The listing builds one solid part. Answer for the finished solid, in the listing's coordinates (mm). A direction names the side the tool comes from. Coordinates: 2 decimals unless noted, no trailing zeros. Order: outer loops, then holes, each group sorted by start corner. A loop starts at its lowest first (then second) coordinate and runs counter-clockwise, first axis right, second up. Notation, with made-up numbers: (57.5, 11) - (69.5, 11) arc R13 cw to (69.5, 19) - close; hole circle Ø3 at (1.5, 43). An arc over 180 degrees is marked (long way). Use one line per item in the form item = value. Start each with the question number.
Item 1: Each of these flat-tipped pins is pushed along its axis until it touches: pin 1 Ø3 at (x, y) = (139.5, 5.5) entering from -Z; pin 2 Ø5 at (x, y) = (48.5, 4.5) entering from -Z; pin 3 Ø4 at (x, z) = (72, 21.5) entering from +Y. Where does it stop, or does it pass through?
Item 2: Section B-B, the plane z = 2 is taken. Write down the section's boundary in (x, y).
Item 3: A tool of negligible diameter and unlimited length cuts with its end or side. For faces 4 (the flat face through (103.68, 5.07, -15)), 5 (the flat face through (137, 5, -21)), 6 (the flat face through (122.249, 5.07, -6.156)), from which of +Z, -Z, +X, -X, +Y, -Y can it reach the whole face along a straight path? Write none if from no direction.
Item 4: Section C-C, the plane x = 119.5 is taken. Write down the section's boundary in (y, z), and give its area (3 significant figures).
Item 5: The mould has two halves that part along Y. Classify faces 1 (the cylindrical face through (75.707, 5.066, 12.856)), 2 (the flat face through (52, 5, -13.966)), 3 (the cylindrical face through (147.846, 1.504, -16.944)): released by +Y, released by -Y, zero draft, split by the parting line, or undercut.
Item 6: Section A-A, the plane x = 138 is taken. Write down the section's boundary in (y, z), and give its area (3 significant figures).
Item 7: Consider line 1 along X through (y, z) = (5.25, 21); line 2 along Z through (x, y) = (81, 2.75); line 3 along Z through (x, y) = (76, 7.25). Determine where each line is inside the solid, lowest interval first. Write a range as [from, to].
from build123d import *

# Parameters (mm, degrees)
RESSALTO_EXTRUS_O1_DEPTH = 10
ESBO_O4_W                = 13
ESBO_O4_H                = 26
CORTE_EXTRUS_O1_DEPTH    = 153.557132499
ESBO_O5_R                = 2
CORTE_EXTRUS_O2_DEPTH    = 160.086317259
ESBO_O6_W                = 27
ESBO_O6_H                = 10
CORTE_EXTRUS_O3_DEPTH    = 20
FILETE1_R                = 5
FILETE2_R                = 5
ESBO_O7_R                = 1.5
CORTE_EXTRUS_O4_DEPTH    = 158.459379965
ESBO_O8_R                = 1.5
CORTE_EXTRUS_O5_DEPTH    = 20
ESBO_O10_W               = 17
ESBO_O10_H               = 7
CORTE_EXTRUS_O8_DEPTH    = 10


with BuildPart() as part:
    # Esboço1 → Ressalto-extrusão1 (new body)
    with BuildSketch(Plane(origin=(0, 0, 0), x_dir=(1, 0, 0), z_dir=(0, 1, 0))):
        Polygon((0, -26), (0, 26), (70.5, 26), (125.272255751, 21), (149.272255751, 21), (149.272255751, -22), (125.272255751, -22), (96.066533251, -28.85753405), (51.077645734, -29.85753405), align=None)
    extrude(amount=RESSALTO_EXTRUS_O1_DEPTH)

    # Esboço4 → Corte-extrusão1 (cut, through all)
    with BuildSketch(Plane(origin=(0, 10, 0), x_dir=(1, 0, 0), z_dir=(0, 1, 0))):
        with Locations((6.5, 0)):
            Rectangle(ESBO_O4_W, ESBO_O4_H)
    extrude(amount=-CORTE_EXTRUS_O1_DEPTH, mode=Mode.SUBTRACT)

    # Esboço2 → Revolução1 (revolve)
    with BuildSketch(Plane.ZY, mode=Mode.PRIVATE) as revolu_o1_sk:
        with BuildLine():
            Line((-27, 5), (-27, 10.5))
            Line((-27, 10.5), (-11.8, 10.5))
            add(Edge.make_bspline(
                [(-11.8, 10.5), (-11.799257972, 9.25000022), (-11, 9)],
                knots=[0, 0, 0, 1, 1, 1], degree=2))
            Line((-11, 9), (11, 9))
            add(Edge.make_bspline(
                [(11.8, 10.5), (11.782356414, 9.025535941), (11, 9)],
                knots=[0, 0, 0, 1, 1, 1], degree=2))
            Line((11.8, 10.5), (27, 10.5))
            Line((27, 10.5), (27, 5))
            Line((27, 5), (-27, 5))
        make_face()
    revolve(revolu_o1_sk.sketch.rotate(Axis((0, 5, -27), (0, 0, 1)), 90), axis=Axis((0, 5, -27), (0, 0, 1)))

    # Esboço5 → Corte-extrusão2 (cut, through all)
    with BuildSketch(Plane.XY.offset(27)):
        with Locations((0, 5)):
            Circle(ESBO_O5_R)
    extrude(amount=-CORTE_EXTRUS_O2_DEPTH, mode=Mode.SUBTRACT)

    # Esboço6 → Corte-extrusão3 (cut)
    with BuildSketch(Plane(origin=(149.272255751, 0, 0), x_dir=(0, 0, -1), z_dir=(1, 0, 0))):
        with Locations((-0.5, 5)):
            Rectangle(ESBO_O6_W, ESBO_O6_H)
    extrude(amount=-CORTE_EXTRUS_O3_DEPTH, mode=Mode.SUBTRACT)

    # Filete1
    filete1_edges = [part.edges().sort_by_distance(p)[0] for p in [
        (149.272255751, 10, 18),
    ]]
    fillet(filete1_edges, radius=FILETE1_R)

    # Filete2
    filete2_edges = [part.edges().sort_by_distance(p)[0] for p in [
        (149.272255751, 0, -17),
        (149.272255751, 10, -17),
        (149.272255751, 0, 18),
    ]]
    fillet(filete2_edges, radius=FILETE2_R - 0.0001)  # a hair under: the kernel refuses the full size

    # Esboço7 → Corte-extrusão4 (cut, through all)
    with BuildSketch(Plane.XY.offset(22)):
        with Locations((144.272255751, 5)):
            Circle(ESBO_O7_R)
    extrude(amount=-CORTE_EXTRUS_O4_DEPTH, mode=Mode.SUBTRACT)

    # Esboço8 → Corte-extrusão5 (cut)
    with BuildSketch(Plane(origin=(0.688560438, 0, 30.977568087), x_dir=(0.9997530559290662, 0, -0.02222222222222223), z_dir=(0.02222222222222223, 0, 0.9997530559290662))):
        with Locations((86.901531655, 5)):
            Circle(ESBO_O8_R)
        with Locations((81.901531655, 5)):
            Circle(ESBO_O8_R)
        with Locations((76.901531655, 5)):
            Circle(ESBO_O8_R)
    extrude(amount=-CORTE_EXTRUS_O5_DEPTH, mode=Mode.SUBTRACT)

    # Esboço10 → Corte-extrusão8 (cut)
    with BuildSketch(Plane(origin=(0, 10, 0), x_dir=(1, 0, 0), z_dir=(0, 1, 0))):
        Polygon((96.066533251, -22.85605202), (66.073941573, -23.522718687), (66.073941573, -16.522718687), (96.066533251, -15.85605202), align=None)
        Polygon((13, 13), (27.658080306, 0), (13, -13), align=None)
        Polygon((14.715215875, 17), (30.605506577, 2.907173735), (33.988145027, 6.721249585), (33.988145027, 17), align=None)
        Polygon((30.605506577, -4.06909346), (15.267814751, -17.67182926), (54.15706585, -20.608859895), align=None)
        Polygon((33.658080306, 0), (42.012333551, 9.419793458), (56.871686456, 9.419793458), (72.605550348, -4.534300553), (72.605550348, -14.178506447), (53.847357844, -14.178506447), align=None)
        with Locations((51.715539775, 17.466082457)):
            Rectangle(ESBO_O10_W, ESBO_O10_H)
        Polygon((85.85936677, 16.625472682), (111.060316292, 3.717254981), (121.012658968, 13.416430831), align=None)
        Polygon((129.272255751, -14), (115.419880228, -0.5), (129.272255751, 13), align=None)
        Polygon((65.215539775, 18.996331638), (65.215539775, 9.387469518), (84.442487674, -7.664580783), (92.451959357, -7.664580783), (100.203174703, 1.075260526), align=None)
        Polygon((115.511410207, -15.047093106), (106.507920849, -6.272633726), (101.066533251, -12.408041141), (101.066533251, -18.438765254), align=None)
    extrude(amount=-CORTE_EXTRUS_O8_DEPTH, mode=Mode.SUBTRACT)


solid = part.part
Response:
q1.pin_1 = -21
q1.pin_2 = -26
q1.pin_3 = 10
q2.outline = circle Ø8 at (0, 5); (25.4, 0) - (36.51, 0) - (36.51, 10) - (25.4, 10) - close; (69.75, 0) - (78.06, 0) - (78.06, 10) - (69.75, 10) - close; (97.48, 0) - (116.96, 0) - (116.96, 10) - (97.48, 10) - close; hole circle Ø4 at (0, 5)
q3.face_4 = +Y, -Y
q3.face_5 = -Z, +X, +Y, -Y
q3.face_6 = +X, +Y, -Y
q4.outline = (0, -21.53) - (10, -21.53) - (10, -13.55) - (0, -13.55) - close; (0, -11.94) - (10, -11.94) - (10, -3.48) - (0, -3.48) - close; (0, 4.48) - (10, 4.48) - (10, 23.36) - (0, 23.36) - close
q4.area = 353 mm2
q5.face_1 = undercut
q5.face_2 = zero draft
q5.face_3 = released by -Y
q6.outline = (0, -21) - (10, -21) - (10, -13) - (0, -13) - close; (0, 14) - (10, 14) - (10, 22) - (0, 22) - close
q6.area = 160 mm2
q7.line_1 = [-5.49, -1.98], [1.98, 66.07], [96.07, 142.79], [145.75, 149.27]
q7.line_2 = [-25.04, -10.91], [4.61, 16.19], [23.19, 29.19]
q7.line_3 = [-25.5, -13.47], [0.18, 16.3], [23.3, 29.3]
